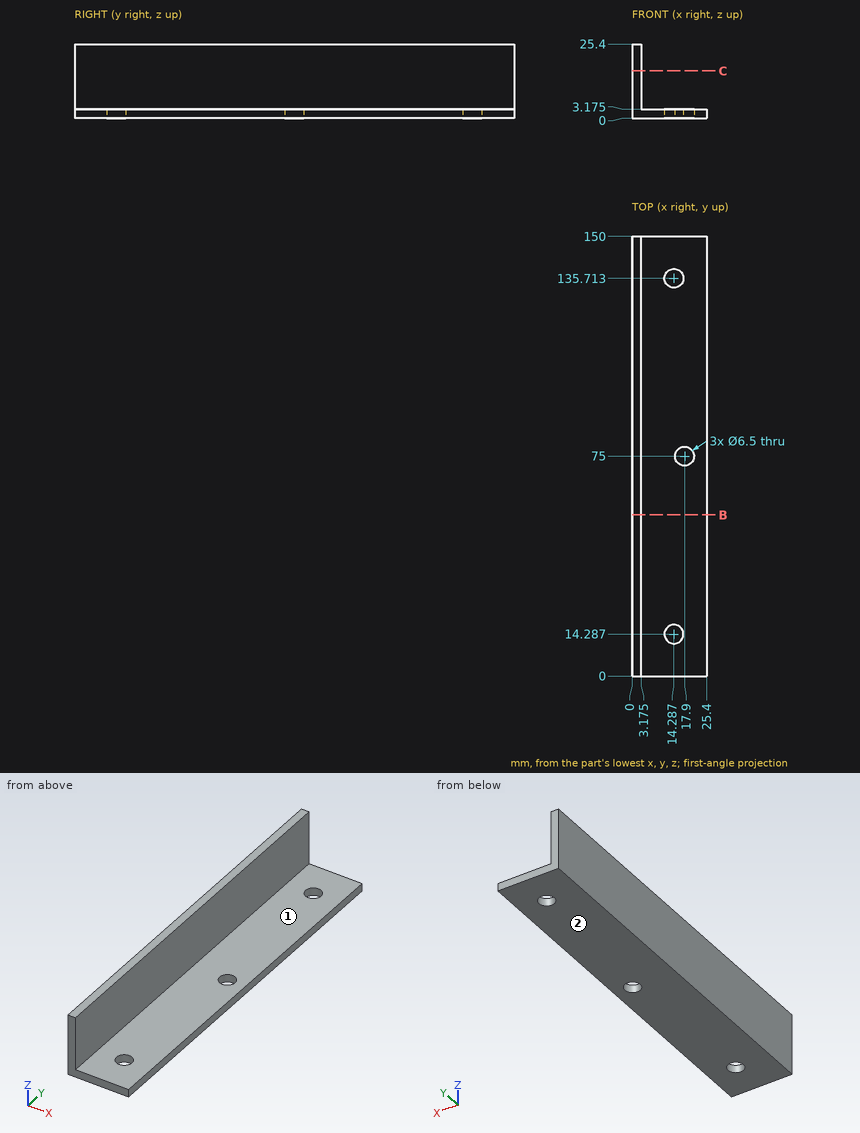
The figure shows three views and two pictorial views of one solid part (mm, origin at its lowest corner). Answer the questions. A direction names the side the tool comes from. Round coordinates to 2 decimals unless told otherwise and drop trailing zeros. Order: outer loops, then holes, each group sorted by start corner. A loop starts at its lowest first (then second) coordinate and runs counter-clockwise, first axis right, second up.
Q1. A cutting plane is placed at C-C, the plane z = 16.25. Determine the outline of the cut face in (x, y) (1 decimal).
Solution:
outline: (0, 0) - (3.2, 0) - (3.2, 150) - (0, 150) - close
Q2. A tool of negligible diameter and unlimited length cuts with its end or side. For the marked faces 1 and 2, from which of +Z, -Z, +X, -X, +Y, -Y can it reach the whole face along a straight path? Write none if from no direction.
Solution:
face 1: +Z, +X, +Y, -Y
face 2: -Z, +X, -X, +Y, -Y
Q3. Find the intervals of material crossed by line 1 along X through (y, z) = (75, 2.25); line 2 along X through (y, z) = (108, 19) (1 decimal), in increasing order.
Solution:
line 1: x = 0 to 14.65, 21.15 to 25.4
line 2: x = 0 to 3.2
Q4. Given pin 1 Ø4 at (y, z) = (133.5, 21.5) entering from +X (1 decimal); pin 2 Ø8.5 at (x, y) = (14.29, 135.71) entering from +Z (1 decimal), each flat-ended and moving along its own axis, determine where each tip first touches the part or whether it passes through.
Solution:
pin 1: stops at x = 3.2
pin 2: stops at z = 3.2
Q5. A cutting plane is placed at B-B, the plane y = 55. Determine the outline of the cut face in (x, z) (1 decimal), then the cut area to 3 significant figures.
Solution:
outline: (0, 0) - (25.4, 0) - (25.4, 3.2) - (3.2, 3.2) - (3.2, 25.4) - (0, 25.4) - close
area: 151 mm2
